Source: three-view drawing plus pictorial views. Frame: mm from the lowest corner of the part. Give positions to 0.01 mm unless a question says otherwise; leave off trailing zeros. Order: outer loops, then holes, each group sorted by start corner. A loop starts at its lowest first (then second) coordinate and runs counter-clockwise, first axis right, second up. Notation, with made-up numbers: M -7.75,-16.75 L 45.25,-16.75 A22 ccw 45.25,10.25 Z; hole C -7.75,-14.75 d8. An arc over 180 degrees is marked long. Use CSV: the item, a comma, the result in double quotes. Start each with the question number.
Item 1: Section query B-B on z = 1.15. Count the separate pieces of the cut face and the enclosed holes in it, and give its area (3 significant figures).
Item 2: Section query A-A on x = 37.5. Return loops of the section in (y, z).
Item 3: Ray query, probe 1 along Y at (x, z) = (53.5, 0.25); probe 2 along Y at (x, z) = (50, 0.35); probe 3 along X at (y, z) = (10, 0.25). Return the intervals inside material, ascending. Write a range as from..to.
Item 4: Section query C-C on x = 51. Return loops of the section in (y, z), and give its area (3 significant figures).
Item 5: Section query D-D on y = 32. Return loops of the section in (x, z).
Item 6: First-contact query: pin 1 (12 mm diameter, centred on x = 68.5, y = 23, fed in from -Z); pin 2 (1 mm diameter, centred on y = 48.5, z = 1, fed in from -X); pin 3 (1 mm diameter, centred on x = 3, z = 1.5, fed in from -Y); pin 4 (0.6 mm diameter, centred on y = 22.5, z = 1, fed in from -X). Flat tips, straight axial feed; report the tip coordinate or a pass-through.
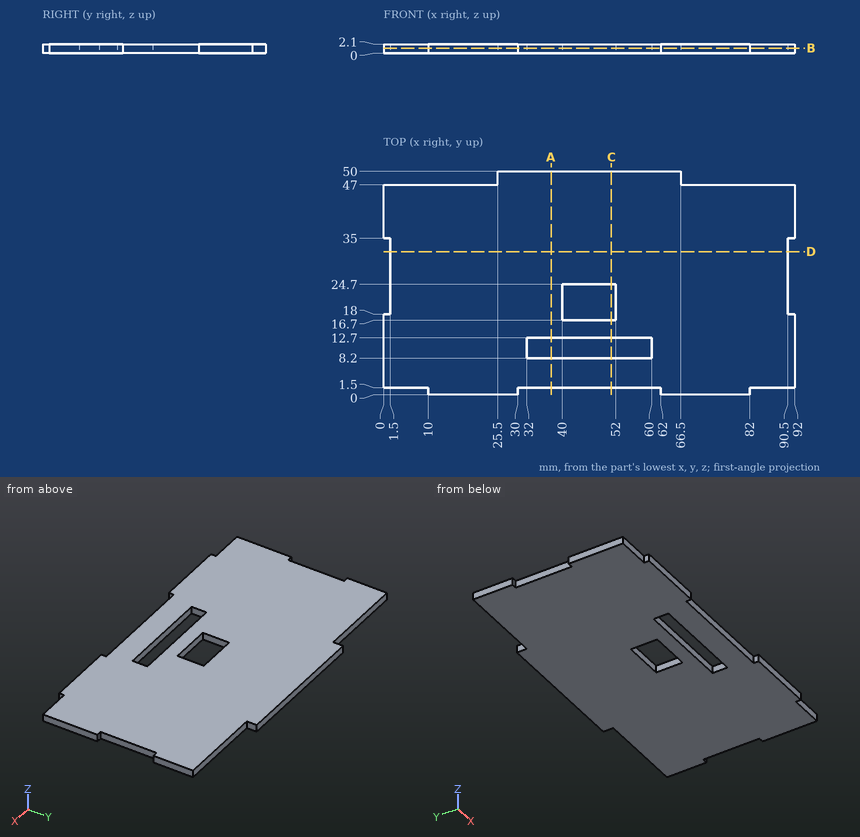
Verdict:
1,separate pieces,"1"
1,enclosed holes,"2"
1,area,"4,100 mm2"
2,outline,"M 1.5,0 L 8.2,0 L 8.2,2.1 L 1.5,2.1 Z; M 12.7,0 L 50,0 L 50,2.1 L 12.7,2.1 Z"
3,probe 1,"1.5..8.2, 12.7..50"
3,probe 2,"1.5..8.2, 12.7..16.7, 24.7..50"
3,probe 3,"0..32, 60..92"
4,outline,"M 1.5,0 L 8.2,0 L 8.2,2.1 L 1.5,2.1 Z; M 12.7,0 L 16.7,0 L 16.7,2.1 L 12.7,2.1 Z; M 24.7,0 L 50,0 L 50,2.1 L 24.7,2.1 Z"
4,area,"75.6 mm2"
5,outline,"M 1.5,0 L 90.5,0 L 90.5,2.1 L 1.5,2.1 Z"
6,pin 1,"z = 0"
6,pin 2,"x = 25.5"
6,pin 3,"y = 1.5"
6,pin 4,"x = 1.5"
